Build history of the part. All positions in model axes, mm. Face numbers are marked on the shaded views. A direction names the side the tool comes from. Give positions to 0.01 mm unless a question says otherwise; leave off trailing zeros. Write each loop counter-clockwise with the first axis right and the second up, starting at its lowest first coordinate (ties: lowest second). Pieces come first, ordered by that corner, then holes. Notation, with made-up numbers: (5, 12) -> (20, 12) arc R13 cw to (20, 17) -> close; hole circle Ø5 at (54.5, 74.5). An arc over 180 degrees is marked (long way). Write item = value, one per line. Start each with the question number.
Q1. Saw through at B-B, the plane y = 0. List the corners of the cut face in (x, z).
Q2. Tool access for the marked faces 1, 2 and 3: list every direction of +Z, -Z, +X, -X, +Y, -Y with a clear straight run to the whole face (end or side of a thin tool).
Q3. Wall check: line 1 (Z direction, x = 95.4, y = 0); line 2 (Z direction, x = 67.5, y = 5); line 3 (Z direction, x = 96, y = 12). Give the ranges that are in metal, low to high.
Q4. Drop flat-ended pins along their axis: P1, Ø5, axis at y = -0.5, z = -2.5, coming from the +X side; P2, Ø1, axis at x = 59, z = 17.5, coming from the -Y side; P3, Ø4, axis at x = 47.5, y = -7.5, coming from the +Z side. Give the stop position or say it passes through.
Q5. Saw through at C-C, the plane x = 24. List the corners of the cut face in (y, z).
Q6. Mould opens along X. For the marked faces 4, 5, 6 and 7 say: pulls with the +X half, pulls with the -X half, needs draft (parallel to the pull), parting line crosses it, or undercut.
from build123d import *

# Parameters (mm, degrees)
CUT_EXTRUDE_1_DEPTH      = 46
CUT_EXTRUDE_1_DEPTH_BACK = 46


with BuildPart() as part:
    # 草圖1 → 旋轉1 (revolve)
    with BuildSketch(Plane.XY):
        with BuildLine():
            Line((6, 8), (49, 8))
            ThreePointArc((49, 8), (53.242640687, 9.757359313), (55, 14))
            Line((55, 14), (55, 37))
            ThreePointArc((55, 37), (57.343145751, 42.656854249), (63, 45))
            Line((63, 45), (97, 45))
            ThreePointArc((97, 45), (102.656854249, 42.656854249), (105, 37))
            Line((105, 37), (105, 28))
            ThreePointArc((105, 28), (102.656854249, 22.343145751), (97, 20))
            Line((97, 20), (95, 20))
            Line((95, 20), (95, 17.876303889))
            Line((95, 17.876303889), (77.395277335, 14.772116295))
            ThreePointArc((77.395277335, 14.772116295), (70.625310141, 11.709619552), (66.155739431, 5.773772537))
            Line((66.155739431, 5.773772537), (75, 5))
            Line((75, 5), (75, 0))
            Line((75, 0), (-10, 0))
            ThreePointArc((-10, 0), (-4.472135955, 8.94427191), (6, 8))
        make_face()
    revolve(axis=Axis((0, 0, 0), (1, 0, 0)))

    # 草圖2 → 除料-伸長1 (cut, two sides)
    with BuildSketch(Plane.XY) as cut_extrude_1_sk:
        with BuildLine():
            Line((-264.793827917, 38.720624717), (-8.660254038, 5))
            Line((-8.660254038, 5), (16.560866404, 1.679576502))
            ThreePointArc((16.560866404, 1.679576502), (18.033815464, 0), (16.560866404, -1.679576502))
            Line((16.560866404, -1.679576502), (-8.660254038, -5))
            Line((-8.660254038, -5), (-264.793827917, -38.720624717))
            Line((-264.793827917, -38.720624717), (-781.481308701, -38.720624717))
            Line((-781.481308701, -38.720624717), (-781.481308701, 38.720624717))
            Line((-781.481308701, 38.720624717), (-264.793827917, 38.720624717))
        make_face()
    extrude(amount=CUT_EXTRUDE_1_DEPTH, mode=Mode.SUBTRACT)
    extrude(cut_extrude_1_sk.sketch, amount=-CUT_EXTRUDE_1_DEPTH_BACK, mode=Mode.SUBTRACT)


solid = part.part
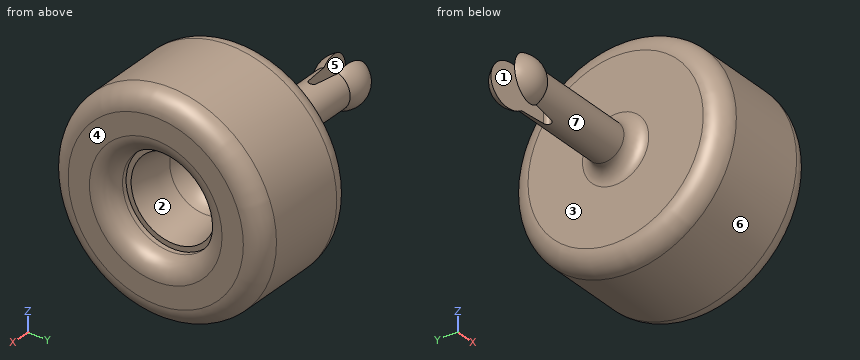
Report:
q1.outline = (18.03, -8) -> (49, -8) arc R6 cw to (55, -14) -> (55, -37) arc R8 ccw to (63, -45) -> (97, -45) arc R8 ccw to (105, -37) -> (105, -28) arc R8 ccw to (97, -20) -> (95, -20) -> (95, -17.88) -> (77.4, -14.77) arc R15 cw to (66.16, -5.77) -> (75, -5) -> (75, 5) -> (66.16, 5.77) arc R15 cw to (77.4, 14.77) -> (95, 17.88) -> (95, 20) -> (97, 20) arc R8 ccw to (105, 28) -> (105, 37) arc R8 ccw to (97, 45) -> (63, 45) arc R8 ccw to (55, 37) -> (55, 14) arc R6 cw to (49, 8) -> (18.03, 8) -> close
q2.face_1 = +Z, -Z, -X
q2.face_2 = +X
q2.face_3 = -X
q3.line_1 = -45 to -20, 20 to 45
q3.line_2 = -44.72 to -6.61, -2.64 to 2.64, 6.61 to 44.72
q3.line_3 = -43.37 to -16, 16 to 43.37
q4.P1 = 75
q4.P2 = -40.66
q4.P3 = 5.81
q5.outline = circle Ø16 at (0, 0)
q6.face_4 = pulls with the +X half
q6.face_5 = pulls with the -X half
q6.face_6 = needs draft
q6.face_7 = undercut
